from build123d import *

# Parameters (mm, degrees)
F2_R     = 5
F3_DEPTH = 27
F4_R     = 2


# Not quite as in the source:
# - a feature names something its author has since deleted; it is built from what else it names


with BuildPart() as f1:
    # F0 (on Right) → F1 (revolve)
    with BuildSketch(Plane.YZ):
        Polygon((-5, -11), (-5, 16), (-45, 16), (-45, 10), (-36.3397459622, 5), (-36.3397459622, 0), (-45, -5), (-45, -11), align=None)
    revolve(axis=Axis((0, 0, -0.4931497392), (0, 0, -1)))

    # F2 (on face) → F3 (cut, through all)
    with BuildSketch(Plane.XY.offset(16)):
        with Locations((-28.5316954889, 9.2705098312)):
            Circle(F2_R)
        with Locations((-17.6335575688, -24.2705098312)):
            Circle(F2_R)
        with Locations((17.6335575688, -24.2705098312)):
            Circle(F2_R)
        with Locations((28.5316954889, 9.2705098312)):
            Circle(F2_R)
        with Locations((0, 30)):
            Circle(F2_R)
    extrude(amount=-F3_DEPTH, mode=Mode.SUBTRACT)

    # F4
    f4_edges = [f1.edges().sort_by_distance(p)[0] for p in [
        (0, 36.339746, 0),
        (0, 36.339746, 5),
    ]]
    fillet(f4_edges, radius=F4_R)


solid = f1.part
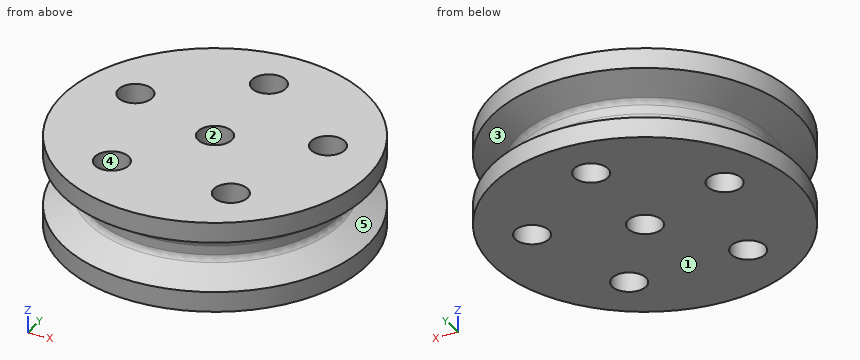
Read the model definition and answer for the solid it produces. Units are mm, in the model's axes. Face numbers are marked on the shaded views. A direction names the side the tool comes from. Give positions to 0.01 mm unless a question says otherwise; leave off trailing zeros. Write each loop counter-clockwise with the first axis right and the second up, starting at its lowest first coordinate (ties: lowest second). Pieces come first, ordered by that corner, then holes. Notation, with made-up numbers: (39.5, 66.5) -> (64.5, 66.5) arc R26 cw to (64.5, 101.5) -> close; hole circle Ø4 at (15, -18.75). An arc over 180 degrees is marked (long way). Answer as a JSON object with one key per item and string values. Group by question number.
1) The mould has two halves that part along Z. Classify the marked faces 1, 2 and 3: +Z half, -Z half, draft (parallel to the pull), parting line (faces both ways), or undercut.
2) Each of these flat-tipped pins is pushed along its axis until it touches: P1, Ø16, axis at x = -28.53, y = 9.27, coming from the -Z side; P2, Ø4, axis at y = 7.5, z = 12.5, coming from the -X side; P3, Ø8, axis at y = -24.5, z = 10.5, coming from the +X side; P4, Ø1, axis at x = -26.5, z = -8, coming from the +Y side. Where does it stop, or does it pass through?
3) Consider L1, parallel to Y at x = -4.5, z = -3.25; L2, parallel to X at y = -26.5, z = 10.5; L3, parallel to Y at x = 0, z = -3. Determine where each line is inside the solid, lowest interval first. Write a range as from..to.
4) Find section B-B (x = 0). Count the separate pieces of the cut face and the enclosed holes in it, and give its area (3 significant figures).
5) Find section A-A (z = -2.25). Write down the section's boundary in (x, y), and give its area (3 significant figures).
6) Find section C-C (z = 7). Write down the section's boundary in (x, y), and give its area (3 significant figures).
7) A tool of negligible diameter and unlimited length cuts with its end or side. For the marked faces 4 and 5, from which of +Z, -Z, +X, -X, +Y, -Y can it reach the whole face along a straight path? Write none if from no direction.
Values follow:
{
 "1": {"face 1": "-Z half", "face 2": "draft", "face 3": "undercut"},
 "2": {"P1": "stops at z = -11", "P2": "stops at x = -44.66", "P3": "stops at x = 40.06", "P4": "stops at y = 36.73"},
 "3": {"L1": "y = -41.73..-2.18, 2.18..27.82, 32.18..41.73", "L2": "x = -36.37..-22.11, -13.16..13.16, 22.11..36.37", "L3": "y = -41.54..-5, 5..25, 35..41.54"},
 "4": {"separate pieces": "3", "enclosed holes": "0", "area": "1,720 mm2"},
 "5": {"outline": "circle Ø80.47 at (0, 0); hole circle Ø10 at (-28.53, 9.27); hole circle Ø10 at (-17.63, -24.27); hole circle Ø10 at (0, 0); hole circle Ø10 at (0, 30); hole circle Ø10 at (17.63, -24.27); hole circle Ø10 at (28.53, 9.27)", "area": "4,620 mm2"},
 "6": {"outline": "circle Ø79.61 at (0, 0); hole circle Ø10 at (-28.53, 9.27); hole circle Ø10 at (-17.63, -24.27); hole circle Ø10 at (0, 0); hole circle Ø10 at (0, 30); hole circle Ø10 at (17.63, -24.27); hole circle Ø10 at (28.53, 9.27)", "area": "4,510 mm2"},
 "7": {"face 4": "+Z, -Z", "face 5": "none"}
}
